from build123d import *

# Parameters (mm, degrees)
BASE_DEPTH       = 3
BULDGESKETCH_W   = 10
BULDGESKETCH_H   = 40
BULDGE_DEPTH     = 4
HOLESSKETCH_R    = 2
HOLES_DEPTH      = 1
HOLES_DEPTH_BACK = 8


with BuildPart() as part:
    # BaseSketch → Base (new body)
    with BuildSketch(Plane(origin=(0, 0, 0), x_dir=(1, 0, 0), z_dir=(0, 1, 0))):
        Polygon((26, -20), (26, -17), (10, -1.5), (10, 1.5), (26, 17), (26, 20), (-26, 20), (-26, -20), align=None)
    extrude(amount=BASE_DEPTH)

    # BuldgeSketch → Buldge (add)
    with BuildSketch(Plane(origin=(0, 3, 0), x_dir=(1, 0, 0), z_dir=(0, 1, 0))):
        with Locations((-8, 0)):
            Rectangle(BULDGESKETCH_W, BULDGESKETCH_H)
    extrude(amount=BULDGE_DEPTH)

    # HolesSketch → Holes (cut, two sides)
    with BuildSketch(Plane.XZ) as holes_sk:
        with Locations((4, 0)):
            Circle(HOLESSKETCH_R)
        with Locations((16.5, -16)):
            Circle(HOLESSKETCH_R)
        with Locations((16.5, 16)):
            Circle(HOLESSKETCH_R)
        with Locations((-18.5, 0)):
            Circle(HOLESSKETCH_R)
    extrude(amount=HOLES_DEPTH, mode=Mode.SUBTRACT)
    extrude(holes_sk.sketch, amount=-HOLES_DEPTH_BACK, mode=Mode.SUBTRACT)


solid = part.part
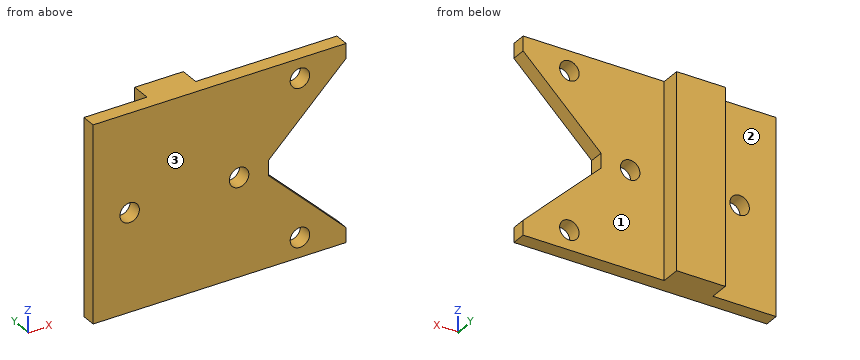
The listing builds one solid part. Answer for the finished solid, in the listing's coordinates (mm). Face numbers are marked on the shaded views. A direction names the side the tool comes from. Coordinates: 2 decimals unless noted, no trailing zeros. Write each loop counter-clockwise with the first axis right and the second up, starting at its lowest first coordinate (ties: lowest second). Pieces come first, ordered by that corner, then holes. Notation, with made-up numbers: M 9,-0.5 L 62,-0.5 A20 cw 62,11.5 Z; hole C -5.75,30 d5. An arc over 180 degrees is marked long. Put each result on its own line as item: value. Start each with the question number.
1. A cutting plane is placed at B-B on z = -16. Write down the section's boundary in (x, y), then the cut area to 3 significant figures.
2. Consider line 1 (Z direction, x = -18.5, y = 1.6); line 2 (Z direction, x = 16.5, y = 1.5); line 3 (X direction, y = 2, z = -1). Determine where each line is inside the solid, lowest interval first. Write a range as from..to.
3. Which of the six approach directions +Z, -Z, +X, -X, +Y, -Y give full straight-line access (tool end or side, diameter ignored) to the marked faces 1, 2 and 3?
4. A cutting plane is placed at A-A on x = 4. Write down the section's boundary in (y, z), then the cut area to 3 significant figures.
5. A cutting plane is placed at C-C on x = 17.5. Write down the section's boundary in (y, z), then the cut area to 3 significant figures.
6. Flat-ended cylindrical pins translate along their axes: P1, Ø5, axis at x = -18.5, z = 0, coming from the -Y side; P2, Ø14.5, axis at x = 13.5, z = 6, coming from the +Y side; P3, Ø2, axis at y = 4.5, z = 6, coming from the -X side; P4, Ø3.5, axis at y = 1, z = 0.5, coming from the +X side. Find the tip coordinate at first contact, or state that the pin passes through.
7. A cutting plane is placed at D-D on z = 8. Write down the section's boundary in (x, y), then the cut area to 3 significant figures.
Resolved:
1. outline: M -26,0 L 14.5,0 L 14.5,3 L -3,3 L -3,7 L -13,7 L -13,3 L -26,3 Z; M 18.5,0 L 24.97,0 L 24.97,3 L 18.5,3 Z
1. area: 181 mm2
2. line 1: z = -20..-2, 2..20
2. line 2: z = -20..-18, -14..-7.8, 7.8..14, 18..20
2. line 3: x = -26..-20.23, -16.77..2.27, 5.73..10
3. face 1: +Z, -Z, +X, +Y
3. face 2: +Z, -Z, -X, +Y
3. face 3: +Z, -Z, +X, -X, -Y
4. outline: M 0,-20 L 3,-20 L 3,-2 L 0,-2 Z; M 0,2 L 3,2 L 3,20 L 0,20 Z
4. area: 108 mm2
5. outline: M 0,-20 L 3,-20 L 3,-17.73 L 0,-17.73 Z; M 0,-14.27 L 3,-14.27 L 3,-8.77 L 0,-8.77 Z; M 0,8.77 L 3,8.77 L 3,14.27 L 0,14.27 Z; M 0,17.73 L 3,17.73 L 3,20 L 0,20 Z
5. area: 46.6 mm2
6. P1: stops at y = 0
6. P2: stops at y = 3
6. P3: stops at x = -13
6. P4: stops at x = 10.77
7. outline: M -26,0 L 16.71,0 L 16.71,3 L -3,3 L -3,7 L -13,7 L -13,3 L -26,3 Z
7. area: 168 mm2
